from build123d import *
from build123d.topology import SkipClean

# Parameters (mm, degrees)
SKETCH1_R           = 4.5
SKETCH1_R_2         = 3
BOSS_EXTRUDE1_DEPTH = 4
SKETCH2_R           = 1
BOSS_EXTRUDE2_DEPTH = 2


with BuildPart() as part:
    # Sketch1 → Boss-Extrude1 (new body)
    with BuildSketch(Plane(origin=(0, 0, 0), x_dir=(1, 0, 0), z_dir=(0, 1, 0))):
        with Locations(Location((0, 0, 0), (0, 0, 270))):
            Circle(SKETCH1_R)
        with Locations(Location((0, 0, 0), (0, 0, 270))):
            Circle(SKETCH1_R_2, mode=Mode.SUBTRACT)
    extrude(amount=BOSS_EXTRUDE1_DEPTH)

    # Sketch2 → Boss-Extrude2 (add)
    with SkipClean():  # the faces are left unmerged after this step: merging them gives an invalid solid
        with BuildSketch(Plane(origin=(0, 4, 0), x_dir=(1, 0, 0), z_dir=(0, 1, 0))):
            with BuildLine():
                Line((-4.453412293, 0.645847467), (-2.226706146, 16))
                ThreePointArc((-2.226706146, 16), (0, 17.927076266), (2.226706146, 16))
                Line((2.226706146, 16), (4.453412293, 0.645847467))
                ThreePointArc((4.453412293, 0.645847467), (0, -4.5), (-4.453412293, 0.645847467))
            make_face()
            with Locations(Location((0, 16, 0), (0, 0, 270))):
                Circle(SKETCH2_R, mode=Mode.SUBTRACT)
        extrude(amount=BOSS_EXTRUDE2_DEPTH)
    add(part.part.scale(1), mode=Mode.REPLACE)  # the faces are merged on a copy


solid = part.part
Work out the finished part from the listing and answer in its coordinate system (mm). A direction names the side the tool comes from. Round coordinates to 2 decimals unless told otherwise and drop trailing zeros. Write each loop counter-clockwise with the first axis right and the second up, starting at its lowest first coordinate (ties: lowest second). Pieces come first, ordered by that corner, then holes. Notation, with made-up numbers: (67, 21.25) - (103, 21.25) arc R20 cw to (103, 25.25) - close; hole circle Ø2 at (-1.75, 73.25). An arc over 180 degrees is marked (long way). Answer in a Markdown table with one row per item. Add a question column.
1. Find the intervals of material crossed by line 1 along X through (y, z) = (4.75, -16); line 2 along X through (y, z) = (1.25, 0); line 3 along Y through (x, z) = (0.5, -10.75), in increasing order. Write a range as from..to.
2. For faces 1 (the flat face through (3.324, 4.986, -8.43)), 2 (the cylindrical face through (0.9, 1.97, 2.86)), determine the directions among +Z, -Z, +X, -X, +Y, -Y from which every point of the face is accessible in a straight line to the end or side of a thin tool.
3. A cutting plane is placed at A-A, the plane x = 0. Determine the outline of the cut face in (y, z), and give its area (3 significant figures).
4. Given pin 1 (2 mm diameter, centred on x = -3.5, y = 2.5, fed in from +Z); pin 2 (2 mm diameter, centred on x = -3, y = 1.5, fed in from -Z); pin 3 (1.5 mm diameter, centred on y = 2, z = -13, fed in from +X); pin 4 (2 mm diameter, centred on x = 3, z = -14.5, fed in from -Y), each flat-ended and moving along its own axis, determine where each tip first touches the part or whether it passes through.
5. A cutting plane is placed at C-C, the plane y = 1. Determine the outline of the cut face in (x, z), and give its area (3 significant figures).
6. The mould has two halves that part along X. Classify faces 3 (the flat face through (0, 4, -9)), 4 (the cylindrical face through (-0.045, 4.986, -17.927)), 5 (the flat face through (0, 4, 0)): +X half, -X half, draft (parallel to the pull), parting line (faces both ways), or undercut.
7. A cutting plane is placed at D-D, the plane z = -10.5. Determine the outline of the cut face in (x, y), and give its area (3 significant figures).
8. A cutting plane is placed at B-B, the plane z = 0. Determine the outline of the cut face in (x, y).
Worked out:
| question | item | result |
|---|---|---|
| 1 | line 1 | -2.23..-1, 1..2.23 |
| 1 | line 2 | -4.5..-3, 3..4.5 |
| 1 | line 3 | 4..6 |
| 2 | face 1 | -Z, +X, +Y, -Y |
| 2 | face 2 | -Y |
| 3 | outline | (0, -4.5) - (4, -4.5) - (4, -15) - (6, -15) - (6, 4.5) - (0, 4.5) - (0, 3) - (4, 3) - (4, -3) - (0, -3) - close; (4, -17.93) - (6, -17.93) - (6, -17) - (4, -17) - close |
| 3 | area | 52.9 mm^2 |
| 4 | pin 1 | z = 3.74 |
| 4 | pin 2 | z = -4.03 |
| 4 | pin 3 | through |
| 4 | pin 4 | y = 4 |
| 5 | outline | circle Ø9 at (0, 0); hole circle Ø6 at (0, 0) |
| 5 | area | 35.3 mm^2 |
| 6 | face 3 | draft |
| 6 | face 4 | parting line |
| 6 | face 5 | undercut |
| 7 | outline | (-3.02, 4) - (3.02, 4) - (3.02, 6) - (-3.02, 6) - close |
| 7 | area | 12.1 mm^2 |
| 8 | outline | (-4.5, 0) - (-3, 0) - (-3, 4) - (3, 4) - (3, 0) - (4.5, 0) - (4.5, 6) - (-4.5, 6) - close |
